Design review of the part built by this model. Coordinates are the model's own, in mm. A direction names the side the tool comes from. Round coordinates to 2 decimals unless told otherwise and drop trailing zeros. Loops run counter-clockwise (first coordinate to the right, second up) from the corner with the lowest first, then second, coordinate; pieces in that order, holes last. Notation, with made-up numbers: (50.5, -33.75) -> (64.5, -33.75) arc R10 ccw to (64.5, -17.75) -> close; hole circle Ø10 at (50, 4.25). An arc over 180 degrees is marked (long way). Answer as CSV lines item,"result". Start each with the question number.
(1) Take a section at C-C, the plane x = 0. Write out the cut boundary in (y, z) (3 decimals), and give its area (3 significant figures).
(2) Take a section at B-B, the plane y = 3.4. Write out the cut boundary in (x, z) (3 decimals).
(3) To check wall thickness, follow line 1 (X direction, y = 4.2, z = 0) (3 decimals); line 2 (Y direction, x = -6, z = -1.25); line 3 (X direction, y = 3.8, z = 3.75). State the ranges of each line that lie inside material, in increasing order. Write a range as from..to.
(4) Take a section at A-A, the plane z = 0. Write out the cut boundary in (x, y) (3 decimals), and give its area (3 significant figures).
(5) Machinability: for faces 1 (the face through (0.379, 3.479, -8.617)), 2 (the face through (9, 5, 0)), which of the approach directions +Z, -Z, +X, -X, +Y, -Y give a long, thin tool a straight path to every point of the face, cutting with its end or side? Answer none if there is none.
(6) Take a section at D-D, the plane y = 1.35. Write out the cut boundary in (x, z), and give its area (3 significant figures).
(7) For P1, Ø1.5, axis at x = -5, y = 4.5, coming from the +Z side; P2, Ø1.5, axis at y = 4.5, z = -2, coming from the +X side; P3, Ø1, axis at x = 4, y = 1, coming from the -Z side, all flat-tipped, find the tip position at first contact; note any pin that passes through.
(8) Draft analysis for pull direction X (two halves, no side actions). For faces 3 (the face through (-6.47, 3.99, -8.43)), 4 (the face through (-4, 2, 4)), 5 (the face through (-3.3, 0, 3.3)), state which applies: +X half, -X half, draft (parallel to the pull), parting line (faces both ways), or undercut.
from build123d import *

# Parameters (mm, degrees)
CROQUIS1_R              = 10.625
CROQUIS1_R_2            = 8.625
SALIENTE_EXTRUIR1_DEPTH = 5
CROQUIS1_3_R            = 8.625
SALIENTE_EXTRUIR2_DEPTH = 2
REDONDEO1_R             = 3


with BuildPart() as part:
    # Croquis1 → Saliente-Extruir1 (new body)
    with BuildSketch(Plane(origin=(0, 0, 0), x_dir=(1, 0, 0), z_dir=(0, 1, 0))):
        with Locations(Location((0, 0, 0), (0, 0, 270))):
            Circle(CROQUIS1_R)
        with Locations(Location((0, 0, 0), (0, 0, 270))):
            Circle(CROQUIS1_R_2, mode=Mode.SUBTRACT)
    extrude(amount=SALIENTE_EXTRUIR1_DEPTH)

    # Croquis1_3 → Saliente-Extruir2 (add)
    with BuildSketch(Plane(origin=(0, 0, 0), x_dir=(1, 0, 0), z_dir=(0, 1, 0))):
        with Locations(Location((0, 0, 0), (0, 0, 270))):
            Circle(CROQUIS1_3_R)
    extrude(amount=SALIENTE_EXTRUIR2_DEPTH)

    # Croquis2 → Cortar-Revoluci_n1 (revolve, cut)
    with BuildSketch(Plane.XY):
        with BuildLine():
            Line((0, 8.15), (0, -2.15))
            ThreePointArc((0, -2.15), (-5.15, 3), (0, 8.15))
        make_face()
    revolve(axis=Axis((0, 8.15, 0), (0, -1, 0)), mode=Mode.SUBTRACT)

    # Redondeo1
    redondeo1_edges = [part.edges().sort_by_distance(p)[0] for p in [
        (0, 0, -10.625),
    ]]
    fillet(redondeo1_edges, radius=REDONDEO1_R)


solid = part.part
The answers:
1,outline,"(0, -7.625) arc R3 ccw to (3, -10.625) -> (5, -10.625) -> (5, -8.625) -> (2, -8.625) -> (2, -5.052) arc R5.15 cw to (0, -4.186) -> close; (0, 4.186) arc R5.15 cw to (2, 5.052) -> (2, 8.625) -> (5, 8.625) -> (5, 10.625) -> (3, 10.625) arc R3 ccw to (0, 7.625) -> close"
1,area,"31.8 mm²"
2,outline,"circle Ø21.25 at (0, 0); hole circle Ø17.25 at (0, 0)"
3,line 1,"-10.625..-8.625, 8.625..10.625"
3,line 2,"0..2"
3,line 3,"-9.94..-7.77, 7.77..9.94"
4,outline,"(-10.625, 3) arc R3 ccw to (-7.625, 0) -> (-4.186, 0) arc R5.15 cw to (-5.052, 2) -> (-8.625, 2) -> (-8.625, 5) -> (-10.625, 5) -> close; (4.186, 0) -> (7.625, 0) arc R3 ccw to (10.625, 3) -> (10.625, 5) -> (8.625, 5) -> (8.625, 2) -> (5.052, 2) arc R5.15 cw to start"
4,area,"31.8 mm²"
5,face 1,"+Y"
5,face 2,"+Z, -Z, +X, -X, +Y"
6,outline,"circle Ø20.26 at (0, 0); hole circle Ø9.76 at (0, 0)"
6,area,"248 mm²"
7,P1,"z = 9.74"
7,P2,"x = 10.55"
7,P3,"z = -9.47"
8,face 3,"parting line"
8,face 4,"undercut"
8,face 5,"draft"
